Part model, mm, in its own coordinate system. Coordinates: 2 decimals unless noted, no trailing zeros. Loops run counter-clockwise (first coordinate to the right, second up) from the corner with the lowest first, then second, coordinate; pieces in that order, holes last. Notation, with made-up numbers: M -37.75,76.5 L -25.75,76.5 A24 ccw -25.75,102.5 Z; hole C 32,-3 d1. An arc over 180 degrees is marked long. Answer as a JSON object with one key per item and string values. Group by question number.
1. Saw through at B-B on y = 211. Write the cut outline in (x, z), then the cut area to 3 significant figures.
2. Mould opens along X. For faces 1 (the face through (0, 231, 0)), 2 (the face through (0, 9.937, 0)), 3 (the face through (21.57, 96.91, 28.13)) say: released by +X, released by -X, zero draft, split by the parting line, or undercut.
3. Drop flat-ended pins along their axis: pin 1 Ø5 at (y, z) = (197, 21) entering from -X; pin 2 Ø1.5 at (x, z) = (-27, 8) entering from -Y; pin 3 Ø2 at (x, z) = (-13.5, 11.5) entering from +Y. Give the stop position or say it passes through.
4. Saw through at A-A on y = 136.5. Write the cut outline in (x, z).
5. Drill centre lines: L1, parallel to X at y = 114, z = 0.5; L2, parallel to X at y = 133, z = 4. Where is each one in solid material? Low to high.
from build123d import *


with BuildPart() as part:
    # Skica1 → Rotovat1 (revolve)
    with BuildSketch(Plane.XY, mode=Mode.PRIVATE) as rotovat1_sk:
        with BuildLine():
            Line((-2, 9.937438845), (0, 9.937438845))
            Line((0, 9.937438845), (0, 231))
            Line((0, 231), (-12.618810271, 231))
            ThreePointArc((-12.618810271, 231), (-12.903232124, 224.440073791), (-13.253405947, 217.883328719))
            ThreePointArc((-13.253405947, 217.883328719), (-15.159184085, 211.33843471), (-19.721855633, 206.273885742))
            ThreePointArc((-19.721855633, 206.273885742), (-31.283356959, 193.057862433), (-35.45, 176))
            Line((-35.45, 176), (-35.45, 20))
            ThreePointArc((-35.45, 20), (-35.094324076, 11.796758267), (-34.029965847, 3.655086334))
            ThreePointArc((-34.029965847, 3.655086334), (-33.114653771, 2.300717404), (-31.494757975, 2.081516571))
            Line((-31.494757975, 2.081516571), (-9.042779517, 8.69573486))
            ThreePointArc((-9.042779517, 8.69573486), (-5.556185927, 9.513946086), (-2, 9.937438845))
        make_face()
    revolve(rotovat1_sk.sketch.rotate(Axis((0, 0, 0), (0, 1, 0)), 270), axis=Axis((0, 0, 0), (0, 1, 0)))


solid = part.part
Outcome:
{
 "1": {"outline": "C 0,0 d30.71", "area": "741 mm²"},
 "2": {"face 1": "zero draft", "face 2": "undercut", "face 3": "split by the parting line"},
 "3": {"pin 1": "stops at x = -23.1", "pin 2": "stops at y = 2.84", "pin 3": "stops at y = 209.04"},
 "4": {"outline": "C 0,0 d70.9"},
 "5": {"L1": "x = -35.45 to 35.45", "L2": "x = -35.22 to 35.22"}
}
